Model file for the job. Use its own axes, mm. Coordinates: 2 decimals unless noted, no trailing zeros. Put each result on its own line as item: value. Start each with the question number.
1. Drop flat-ended pins along their axis: P1, Ø1, axis at y = 4, z = 1237.5, coming from the -X side; P2, Ø3, axis at x = 0, z = 1294.5, coming from the +Y side; P3, Ø1.5, axis at x = 6, y = 1, coming from the +Z side; P4, Ø1, axis at y = -24.5, z = 1052.5, coming from the +X side. Give the stop position or say it passes through.
2. Drill centre lines: L1, parallel to X at y = -16.5, z = 1642; L2, parallel to Y at x = 0, z = 518.5; L3, parallel to Y at x = -7.5, z = 1018. Where is each one in solid material? Low to high. Write a range as from..to.
3. Saw through at A-A, the plane z = 1332.5. Give the number of separate pieces and of enclosed holes in the cut face, plus the area to 3 significant figures.
```python
from build123d import *

# Parameters (mm, degrees)
SKETCH1_R            = 2.1
BOSS_EXTRUDE2_DEPTH  = 1800
CUT_EXTRUDE1_DEPTH   = 1801
FILLET1_R            = 0.25
FILLET1_OF_MIRROR1_R = 0.25


with BuildPart() as part:
    # Sketch1 → Boss-Extrude2 (new body)
    with BuildSketch(Plane.XY):
        Polygon((8.199993721, -10), (9.999993721, -10), (9.999993721, -4.63999575), (8.199993721, -2.84), (8.199993721, -5.800653822), (6.861313026, -5.800653822), (3.900652213, -2.84), (3.900652213, 2.84), (6.559993721, 5.499347787), (8.199993721, 5.499347787), (8.199993721, 2.84), (9.999993721, 4.64000425), (9.999993721, 10), (4.63999575, 10), (2.84, 8.2), (5.499325592, 8.2), (5.499325592, 6.56), (2.84, 3.900668129), (-2.84, 3.900668129), (-5.49933815, 6.56), (-5.49933815, 8.2), (-2.84, 8.2), (-4.64000425, 10), (-10.000006279, 10), (-10.000006279, 4.63999575), (-8.200006279, 2.84), (-8.200006279, 5.499347787), (-6.560006279, 5.499347787), (-3.900652213, 2.84), (-3.900652213, -2.84), (-6.861299044, -5.800653822), (-8.200006279, -5.800653822), (-8.200006279, -2.84), (-10.000006279, -4.64000425), (-10.000006279, -10), (-8.200006279, -10), (-8.200006279, -7.300653822), (-6.239977665, -7.300653822), (-2.84, -3.900668129), (2.84, -3.900668129), (6.239993721, -7.300653822), (8.199993721, -7.300653822), align=None)
        Circle(SKETCH1_R, mode=Mode.SUBTRACT)
    boss_extrude2 = extrude(amount=BOSS_EXTRUDE2_DEPTH)

    # Sketch2 → Cut-Extrude1 (cut, through all)
    with BuildSketch(Plane.XY.offset(1800)):
        Polygon((-8.200006279, 6.569347787), (-8.200006279, 8.2), (-6.56933815, 8.2), (-6.56933815, 7.630009211), (-7.62999707, 6.569347787), align=None)
        Polygon((8.199993721, 8.2), (8.199993721, 6.569347787), (7.629987016, 6.569347787), (6.569325592, 7.630006706), (6.569325592, 8.2), align=None)
    cut_extrude1 = extrude(amount=-CUT_EXTRUDE1_DEPTH, mode=Mode.SUBTRACT)

    # Fillet1
    fillet1_edges = [part.edges().sort_by_distance(p)[0] for p in [
        (9.999993721, -4.63999575, 900),
        (-10.000006279, -4.64000425, 900),
        (-8.200006279, -2.84, 900),
        (-8.200006279, 2.84, 900),
        (-10.000006279, 4.63999575, 900),
        (-10.000006279, 10, 900),
        (-4.64000425, 10, 900),
        (-2.84, 8.2, 900),
        (2.84, 8.2, 900),
        (4.63999575, 10, 900),
        (9.999993721, 10, 900),
        (9.999993721, 4.64000425, 900),
        (8.199993721, 2.84, 900),
        (8.199993721, -2.84, 900),
    ]]
    fillet(fillet1_edges, radius=FILLET1_R)

    # Mirror1: Boss-Extrude2 across plane
    add(boss_extrude2.mirror(Plane(origin=(0, -10, 0), x_dir=(0, 0, 1), z_dir=(0, -1, 0))))

    # Fillet1 of Mirror1
    fillet1_of_mirror1_edges = [part.edges().sort_by_distance(p)[0] for p in [
        (9.999993721, -15.36000425, 900),
        (-10.000006279, -15.35999575, 900),
        (-8.200006279, -17.16, 900),
        (-8.200006279, -22.84, 900),
        (-10.000006279, -24.63999575, 900),
        (-10.000006279, -30, 900),
        (-4.64000425, -30, 900),
        (-2.84, -28.2, 900),
        (2.84, -28.2, 900),
        (4.63999575, -30, 900),
        (9.999993721, -30, 900),
        (9.999993721, -24.64000425, 900),
        (8.199993721, -22.84, 900),
        (8.199993721, -17.16, 900),
    ]]
    fillet(fillet1_of_mirror1_edges, radius=FILLET1_OF_MIRROR1_R)

    # Mirror2: Cut-Extrude1 across plane
    add(cut_extrude1.mirror(Plane(origin=(0, -10, 0), x_dir=(0, 0, 1), z_dir=(0, -1, 0))), mode=Mode.SUBTRACT)


solid = part.part
```
Final values:
1. P1: stops at x = -9.86
1. P2: stops at y = 3.9
1. P3: passes through
1. P4: stops at x = 10
2. L1: x = -8.86..-8.2, -4.56..4.56, 8.2..8.86
2. L2: y = -23.9..-22.1, -17.9..-16.1, -3.9..-2.1, 2.1..3.9
2. L3: y = -30..-28.2, -26.7..-25.5, -14.2..-12.7, -7.3..-5.8, 5.5..6.7, 8.2..10
3. separate pieces: 1
3. enclosed holes: 7
3. area: 289 mm²
